from build123d import *

# Parameters (mm, degrees)
SCHIZZO1_R                   = 15.25
SCHIZZO1_R_2                 = 10.25
ESTRUSIONE_ESTRUSIONE1_DEPTH = 30
SCHIZZO4_W                   = 15
SCHIZZO4_H                   = 15
ESTRUSIONE_ESTRUSIONE2_DEPTH = 30
SCHIZZO5_W                   = 5
SCHIZZO5_H                   = 15.257950375
TAGLIO_ESTRUSIONE1_DEPTH     = 30
ESTRUSIONE_ESTRUSIONE3_DEPTH = 30
ESTRUSIONE_ESTRUSIONE4_START = 5
ESTRUSIONE_ESTRUSIONE4_DEPTH = 5


with BuildPart() as part:
    # Schizzo1 → Estrusione-Estrusione1 (new body)
    with BuildSketch(Plane(origin=(0, 0, 0), x_dir=(1, 0, 0), z_dir=(0, 1, 0))):
        with Locations(Location((0, 0, 0), (0, 0, 270))):
            Circle(SCHIZZO1_R)
        with Locations(Location((0, 0, 0), (0, 0, 270))):
            Circle(SCHIZZO1_R_2, mode=Mode.SUBTRACT)
    extrude(amount=ESTRUSIONE_ESTRUSIONE1_DEPTH)

    # Schizzo4 → Estrusione-Estrusione2 (add)
    with BuildSketch(Plane.XZ):
        with Locations((0, -17.75)):
            Rectangle(SCHIZZO4_W, SCHIZZO4_H)
    extrude(amount=-ESTRUSIONE_ESTRUSIONE2_DEPTH)

    # Schizzo5 → Taglio-Estrusione1 (cut)
    with BuildSketch(Plane.XZ):
        with Locations((0, -17.621024812)):
            Rectangle(SCHIZZO5_W, SCHIZZO5_H)
    extrude(amount=-TAGLIO_ESTRUSIONE1_DEPTH, mode=Mode.SUBTRACT)

    # Schizzo6 → Estrusione-Estrusione3 (add, through all)
    with BuildSketch(Plane(origin=(0, 30, 0), x_dir=(1, 0, 0), z_dir=(0, 1, 0))):
        with BuildLine():
            Line((3, -15.25), (15, -15.25))
            Line((15, -15.25), (15, -2.75))
            ThreePointArc((15, -2.75), (0, -15.25), (-15, -2.75))
            Line((-15, -2.75), (-15, -15.25))
            Line((-15, -15.25), (-3, -15.25))
            Line((-3, -15.25), (-3, -15.85))
            Line((-3, -15.85), (-7, -21.25))
            Line((-7, -21.25), (-7, -22.25))
            Line((-7, -22.25), (7, -22.25))
            Line((7, -22.25), (7, -21.25))
            Line((7, -21.25), (3, -15.85))
            Line((3, -15.85), (3, -15.25))
        make_face()
    extrude(amount=-ESTRUSIONE_ESTRUSIONE3_DEPTH)

    # Schizzo7 → Estrusione-Estrusione4 (add)
    with BuildSketch(Plane.XZ.offset(ESTRUSIONE_ESTRUSIONE4_START)):
        with BuildLine():
            Line((-15, 15.25), (15, 15.25))
            Line((15, 15.25), (15, 2.75))
            ThreePointArc((15, 2.75), (13.812634565, -6.463251997), (7.5, -13.278271725))
            Line((7.5, -13.278271725), (7.5, -25.25))
            Line((7.5, -25.25), (2.5, -25.25))
            Line((2.5, -25.25), (2.5, -9.992049625))
            ThreePointArc((2.5, -9.992049625), (0, 10.25), (-2.5, -9.992049625))
            Line((-2.5, -9.992049625), (-2.5, -25.25))
            Line((-2.5, -25.25), (-7.5, -25.25))
            Line((-7.5, -25.25), (-7.5, -13.278271725))
            ThreePointArc((-7.5, -13.278271725), (-13.812634565, -6.463251997), (-15, 2.75))
            Line((-15, 2.75), (-15, 15.25))
        make_face()
    extrude(amount=-ESTRUSIONE_ESTRUSIONE4_DEPTH)


solid = part.part
Could you check a few things on this model? Use its own coordinates, in mm. A direction names the side the tool comes from. Coordinates: 2 decimals unless noted, no trailing zeros. Order: outer loops, then holes, each group sorted by start corner. A loop starts at its lowest first (then second) coordinate and runs counter-clockwise, first axis right, second up.
Q1. Thinking about a two-plate mould opening in X: for faces 5 (the cylindrical face through (0.42, -2.54, 10.24)), 6 (the flat face through (-7.5, 12, -19)), 7 (the flat face through (-5, 12, -25.25)), which applies, released by +X, released by -X, zero draft, split by the parting line, or undercut?
Q2. Suppose I cut it at D-D on y = 26.5. Please give me the cut outline in (x, z).
Q3. Please list where these lines run through material, in increasing order: L1, parallel to X at y = 1, z = -14; L2, parallel to X at y = 15.25, z = 0; L3, parallel to Z at x = 5, y = 24.5.
Q4. Which directions (+Z, -Z, +X, -X, +Y, -Y) give clear straight access to the entire face, cutting with the end or side of a thin tool? Please do faces 1 (the flat face through (0, 0, 20)), 2 (the flat face through (-7, 15, 22)), 3 (the flat face through (-4.97, 15.21, 18.51)), 4 (the flat face through (7, 15, 22)).
Q5. Will these pins go through, and if not, where does the flat tip stop? pin 1 (12 mm diameter, centred on y = 18.5, z = -16.5, fed in from +X); pin 2 (6 mm diameter, centred on y = 18, z = 10, fed in from -X); pin 3 (2 mm diameter, centred on x = 3.5, z = 20, fed in from -Y).
Q6. Suppose I cut it at A-A on y = -2. Please give me the cut outline in (x, z), and give its area (3 significant figures).
Answer:
1. face 5: undercut
1. face 6: released by -X
1. face 7: zero draft
2. outline: (-15, 2.75) arc R15.25 ccw to (-7.5, -13.28) - (-7.5, -25.25) - (-2.5, -25.25) - (-2.5, -9.99) - (-2.29, -9.99) arc R10.25 cw (long way) to (2.29, -9.99) - (2.5, -9.99) - (2.5, -25.25) - (7.5, -25.25) - (7.5, -13.28) arc R15.25 ccw to (15, 2.75) - (15, 15.25) - (3, 15.25) - (3, 15.85) - (7, 21.25) - (7, 22.25) - (-7, 22.25) - (-7, 21.25) - (-3, 15.85) - (-3, 15.25) - (-15, 15.25) - close
3. L1: x = -7.5 to -2.5, 2.5 to 7.5
3. L2: x = -15.25 to -10.25, 10.25 to 15.25
3. L3: z = -25.25 to -8.95, 8.95 to 15.25, 18.55 to 22.25
4. face 1: +Z, +X, -X, -Y
4. face 2: +Z, -X, +Y, -Y
4. face 3: -X, +Y, -Y
4. face 4: +Z, +X, +Y, -Y
5. pin 1: stops at x = 11.06
5. pin 2: stops at x = -15
5. pin 3: stops at y = 0
6. outline: (-15, 2.75) arc R15.25 ccw to (-7.5, -13.28) - (-7.5, -25.25) - (-2.5, -25.25) - (-2.5, -9.99) arc R10.28 cw (long way) to (2.5, -9.99) - (2.5, -25.25) - (7.5, -25.25) - (7.5, -13.28) arc R15.25 ccw to (15, 2.75) - (15, 15.25) - (-15, 15.25) - close
6. area: 576 mm2
